Here's the drawing with two shaded views (mm, measured from the low corner). I have some questions. A direction names the side the tool comes from. Round coordinates to 2 decimals unless told otherwise and drop trailing zeros. Loops run counter-clockwise (first coordinate to the right, second up) from the corner with the lowest first, then second, coordinate; pieces in that order, holes last. Notation, with made-up numbers: M 73.5,31 L 88.5,31 A33 cw 88.5,70 Z; hole C 81,-14 d1. An arc over 180 degrees is marked long. Answer as CSV lines item,"result".
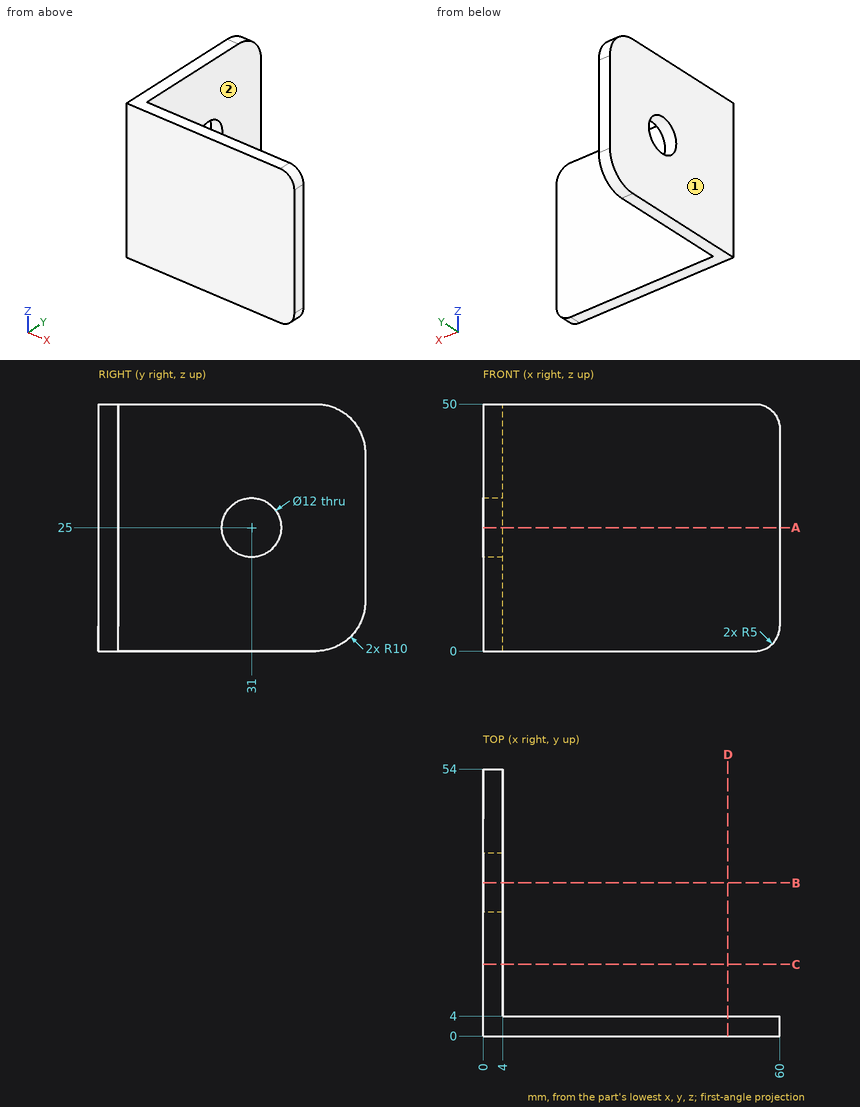
1. I want a section at A-A, the plane z = 25. Please give me the cut outline in (x, y).
Evaluation:
outline,"M 0,0 L 60,0 L 60,4 L 4,4 L 4,25 L 0,25 Z; M 0,37 L 4,37 L 4,54 L 0,54 Z"
2. If I drill on line 1 (X direction, y = 35, z = 9.5); line 2 (Y direction, x = 1, z = 25), over which ranges is the centre line in solid material (lowest first)? Write a range as [from, to].
Evaluation:
line 1,"x = [0, 4]"
line 2,"y = [0, 25], [37, 54]"
3. Which directions (+Z, -Z, +X, -X, +Y, -Y) give clear straight access to the entire face, cutting with the end or side of a thin tool? Please do the marked faces 1 and 2.
Evaluation:
face 1,"+Z, -Z, -X, +Y, -Y"
face 2,"+Z, -Z, +X, +Y"
4. I want a section at B-B, the plane y = 31. Please give me the cut outline in (x, z).
Evaluation:
outline,"M 0,0 L 4,0 L 4,19 L 0,19 Z; M 0,31 L 4,31 L 4,50 L 0,50 Z"
5. I want a section at C-C, the plane y = 14.5. Please give me the cut outline in (x, z).
Evaluation:
outline,"M 0,0 L 4,0 L 4,50 L 0,50 Z"
6. For P1, Ø8, axis at y = 29, z = 34.5, coming from the +X side; P2, Ø9.5, axis at y = 31, z = 25, coming from the +X side, each with a flat end and sliding along its axis, tell me the tip position at first contact or that it passes through.
Evaluation:
P1,"stops at x = 4"
P2,"passes through"
